from build123d import *

# Parameters (mm, degrees)
F1_DEPTH = 15


# Not quite as in the source:
# - ends of sketch curves that miss each other by under 0.0002 mm in the source are joined


with BuildPart() as f1:
    # F0 (on Right) → F1 (new body)
    with BuildSketch(Plane.YZ):
        Polygon((73.9477990592, 7), (117.1341684366, 0), (117.1341684366, 22), (109.1341684366, 22), (109.1341684366, 7), align=None)
        Polygon((-129.6450851485, 0), (117.1341684366, 0), (73.9477990592, 7), (-93.3098772168, 7), (-103.3098761737, 7), (-113.3098740876, 7), (-123.3098730445, 7), (-129.6450851485, 7), align=None)
        Polygon((-129.6450851485, 40), (73.9477990592, 7), (109.1341684366, 7), (-137.6450851485, 47), (-137.6450851485, 0), (-129.6450851485, 0), (-129.6450851485, 7), align=None)
        Polygon((-123.3098730445, 14), (-123.3098730445, 7), (-113.3098740876, 7), (-113.3098730445, 14), (-116.3098730445, 14), (-116.3098730445, 12), (-114.8098730445, 12), (-114.8098730445, 9), (-121.8098730445, 9), (-121.8098730445, 12), (-120.3098730445, 12), (-120.3098730445, 14), align=None)
        Polygon((-113.3098740876, 7), (-103.3098761737, 7), (-103.3098751307, 14), (-106.3098751307, 14), (-106.3098751307, 12), (-104.8098751307, 12), (-104.8098751307, 9), (-111.8098751307, 9), (-111.8098751307, 12), (-110.3098751307, 12), (-110.3098751307, 14), (-113.3098751307, 14), align=None)
        Polygon((-103.3098761737, 7), (-93.3098772168, 7), (-93.3098772168, 14), (-96.3098772168, 14), (-96.3098772168, 12), (-94.8098772168, 12), (-94.8098772168, 9), (-101.8098772168, 9), (-101.8098772168, 12), (-100.3098772168, 12), (-100.3098772168, 14), (-103.3098772168, 14), align=None)
    extrude(amount=F1_DEPTH)


solid = f1.part
Source: CAD feature listing. Evaluate the final solid. Frame: model axes, mm. A direction names the side the tool comes from. Coordinates: 2 decimals unless noted, no trailing zeros. Loops run counter-clockwise (first coordinate to the right, second up) from the corner with the lowest first, then second, coordinate; pieces in that order, holes last. Notation, with made-up numbers: (46.5, 42) - (102.5, 42) arc R26 ccw to (102.5, 61) - close; hole circle Ø5 at (65, 17.25). An arc over 180 degrees is marked (long way). One line per item, written item: value. Start each with the question number.
1. Section A-A (z = 35). Return the cut outline in (x, y).
2. Section B-B (y = 30.5). Return the cut outline in (x, z), and give its area (3 significant figures).
3. Section D-D (y = 91). Return the cut outline in (x, z), and give its area (3 significant figures).
4. Section C-C (z = 18). Return the cut outline in (x, y).
5. Set-up query: faces 1 (the flat face through (15, -30, 6)), 2 (the flat face through (7, 109.134, 15)), 3 (the flat face through (7, -108, 9)), 4 (the flat face through (7, 113, 22)), 5 (the flat face through (7, 117.134, 11)). Return all of +Z, -Z, +X, -X, +Y, -Y with unobstructed straight access to the full face (end or side cutting, diameter ignored); none if empty.
6. Ray query, L1, parallel to Z at x = 2.5, y = 8.5; L2, parallel to Z at x = 12.5, y = -40; L3, parallel to Z at x = 11.25, y = 81. Return the intervals inside material, ascending.
7. Mould query, pull axis Z, two halves, no side actions, for faces 6 (the flat face through (7, -113, 14)), 7 (the flat face through (7, -137.645, 24)), 8 (the flat face through (7.4, -12.53, 26.72)). Classes: pulls with the +Z half, pulls with the -Z half, needs draft (parallel to the pull), parting line crosses it, or undercut.
8. Contact query for flat-ended pins moving along their axis: P1, Ø2.5, axis at x = 6, y = 112.5, coming from the +Z side; P2, Ø0.9, axis at x = 6, y = -94.5, coming from the +Z side; P3, Ø5, axis at x = 10.5, y = -103.5, coming from the +Z side; P4, Ø1.5, axis at y = 70, z = 14.5, coming from the -X side. Output: stop coordinate, or through.
Verdict:
1. outline: (0, -137.65) - (15, -137.65) - (15, -129.65) - (0, -129.65) - close; (0, -98.8) - (15, -98.8) - (15, -63.61) - (0, -63.61) - close
2. outline: (0, 0) - (15, 0) - (15, 7) - (0, 7) - close; (0, 14.04) - (15, 14.04) - (15, 19.75) - (0, 19.75) - close
2. area: 191 mm2
3. outline: (0, 0) - (15, 0) - (15, 9.94) - (0, 9.94) - close
3. area: 149 mm2
4. outline: (0, -137.65) - (15, -137.65) - (15, -129.65) - (0, -129.65) - close; (0, 6.08) - (15, 6.08) - (15, 41.27) - (0, 41.27) - close; (0, 109.13) - (15, 109.13) - (15, 117.13) - (0, 117.13) - close
5. face 1: +Z, -Z, +X, +Y, -Y
5. face 2: +Z, +X, -X
5. face 3: +X, -X
5. face 4: +Z, +X, -X, +Y
5. face 5: +Z, -Z, +X, -X, +Y
6. L1: z = 0 to 7, 17.61 to 23.31
6. L2: z = 0 to 7, 25.47 to 31.17
6. L3: z = 0 to 11.56
7. face 6: undercut
7. face 7: needs draft
7. face 8: pulls with the +Z half
8. P1: stops at z = 22
8. P2: stops at z = 40.08
8. P3: stops at z = 41.87
8. P4: passes through
